from build123d import *

# Parameters (mm, degrees)
SKETCH1_W                      = 63.5
SKETCH1_H                      = 63.5
BOSS_EXTRUDE1_DEPTH            = 31.75
SKETCH2_W                      = 63.5
SKETCH2_H                      = 63.5
SKETCH2_W_2                    = 57.15
SKETCH2_H_2                    = 57.15
BOSS_EXTRUDE2_DEPTH            = 82.55
SKETCH3_W                      = 63.5
SKETCH3_H                      = 12.7
BOSS_EXTRUDE3_DEPTH            = 19.05
F_1_1_DIAMETER_HOLE2_D         = 25.4
F_1_1_DIAMETER_HOLE2_DEPTH     = 63.5
F_1_2_0_5_DIAMETER_HOLE1_D     = 12.7
F_1_2_0_5_DIAMETER_HOLE1_DEPTH = 12.7


with BuildPart() as part:
    # Sketch1 → Boss-Extrude1 (new body)
    with BuildSketch(Plane(origin=(0, 0, 0), x_dir=(1, 0, 0), z_dir=(0, 1, 0))):
        with Locations((31.75, 31.75)):
            Rectangle(SKETCH1_W, SKETCH1_H)
    extrude(amount=BOSS_EXTRUDE1_DEPTH)

    # Sketch2 → Boss-Extrude2 (add)
    with BuildSketch(Plane(origin=(0, 31.75, 0), x_dir=(1, 0, 0), z_dir=(0, 1, 0))):
        with Locations((31.75, 31.75)):
            Rectangle(SKETCH2_W, SKETCH2_H)
        with Locations((31.75, 31.75)):
            Rectangle(SKETCH2_W_2, SKETCH2_H_2, mode=Mode.SUBTRACT)
    extrude(amount=BOSS_EXTRUDE2_DEPTH)

    # Sketch3 → Boss-Extrude3 (add)
    with BuildSketch(Plane(origin=(63.5, 0, 0), x_dir=(0, 0, -1), z_dir=(1, 0, 0))):
        with Locations((31.75, 107.95)):
            Rectangle(SKETCH3_W, SKETCH3_H)
    boss_extrude3 = extrude(amount=BOSS_EXTRUDE3_DEPTH)

    # Mirror2: Boss-Extrude3 across plane
    add(boss_extrude3.mirror(Plane(origin=(31.75, 0, 0), x_dir=(0, 0, 1), z_dir=(1, 0, 0))))

    # 1 (1) Diameter Hole2
    with Locations(Plane(origin=(63.5, 0, 0), x_dir=(0, 0, -1), z_dir=(1, 0, 0))):
        with Locations((31.75, 15.875)):
            Hole(F_1_1_DIAMETER_HOLE2_D / 2, depth=F_1_1_DIAMETER_HOLE2_DEPTH)

    # 1/2 (0.5) Diameter Hole1
    with Locations(Plane(origin=(0, 114.3, 0), x_dir=(1, 0, 0), z_dir=(0, 1, 0))):
        with Locations((72.39, 31.75), (-8.89, 31.593283178)):
            Hole(F_1_2_0_5_DIAMETER_HOLE1_D / 2, depth=F_1_2_0_5_DIAMETER_HOLE1_DEPTH)


solid = part.part
Can you work these out from the model? Positions are in its coordinate system, mm. A direction names the side the tool comes from. Coordinates: 2 decimals unless noted, no trailing zeros. Write each loop counter-clockwise with the first axis right and the second up, starting at its lowest first coordinate (ties: lowest second). Pieces come first, ordered by that corner, then holes. Notation, with made-up numbers: (-27.75, 52) -> (2.25, 52) arc R34 cw to (2.25, 86) -> close; hole circle Ø8 at (69, -33). An arc over 180 degrees is marked (long way). Write item = value, one per line.
(1) For pin 1 (17 mm diameter, centred on y = 72.5, z = -42, fed in from +X); pin 2 (6 mm diameter, centred on x = 23, z = -37, fed in from -Y); pin 3 (9.5 mm diameter, centred on x = 76, z = -23, fed in from -Y); pin 4 (17 mm diameter, centred on y = 70, z = -39.5, fed in from -X), each with a flat end and sliding along its axis, tell me the tip position at first contact or that it passes through.
Verdict:
pin_1 = 63.5
pin_2 = 0
pin_3 = 101.6
pin_4 = 0
(2) If I drill on probe 1 along X at (y, z) = (47, -22) (3 decimals); probe 2 along Z at (x, y) = (72, 108); probe 3 along Z at (x, y) = (-8.89, 110.5), over which ranges is the centre line in solid material (lowest first)?
Verdict:
probe_1 = 0 to 3.175, 60.325 to 63.5
probe_2 = -63.5 to -38.09, -25.41 to 0
probe_3 = -63.5 to -37.94, -25.24 to 0
(3) Imagine slicing it at B-B (z = -49.5). Please give me the cut outline in (x, y) (3 decimals).
Verdict:
outline = (-19.05, 101.6) -> (0, 101.6) -> (0, 0) -> (63.5, 0) -> (63.5, 101.6) -> (82.55, 101.6) -> (82.55, 114.3) -> (60.325, 114.3) -> (60.325, 31.75) -> (3.175, 31.75) -> (3.175, 114.3) -> (-19.05, 114.3) -> close
(4) Imagine slicing it at A-A (x = -8.89). Please give me the cut outline in (y, z).
Verdict:
outline = (101.6, -63.5) -> (114.3, -63.5) -> (114.3, -37.94) -> (101.6, -37.94) -> close; (101.6, -25.24) -> (114.3, -25.24) -> (114.3, 0) -> (101.6, 0) -> close
(5) Thinking about a two-plate mould opening in X: for faces 1 (the face through (-7.513, 107.861, -25.394)), 2 (the face through (63.5, 50, -31)), 3 (the face through (-16, 101.6, -31)), which applies, +X half, -X half, draft (parallel to the pull), parting line (faces both ways), or undercut?
Verdict:
face_1 = undercut
face_2 = +X half
face_3 = draft
(6) On a 3-axis mill with a long thin cutter (end or side, diameter ignored), from which of +Z, -Z, +X, -X, +Y, -Y can I reach the whole of each face in a straight line? I mean faces 4 (the face through (79, 101.6, -31)), 5 (the face through (0, 50, -31)), 6 (the face through (31, 0, -32)), 7 (the face through (78.734, 107.861, -32.029)), 8 (the face through (3.175, 72, -31)). Say none if no direction works.
Verdict:
face_4 = +Z, -Z, +X, -Y
face_5 = +Z, -Z, -X, -Y
face_6 = +Z, -Z, +X, -X, -Y
face_7 = +Y, -Y
face_8 = +Y
(7) Imagine slicing it at D-D (x = 28.5). Please give me the cut outline in (y, z) (3 decimals).
Verdict:
outline = (0, -63.5) -> (114.3, -63.5) -> (114.3, -60.325) -> (31.75, -60.325) -> (31.75, -3.175) -> (114.3, -3.175) -> (114.3, 0) -> (0, 0) -> close; hole circle Ø25.4 at (15.875, -31.75)
(8) Imagine slicing it at C-C (z = -29.5). Please give me the cut outline in (x, y) (3 decimals), and give its area (3 significant figures).
Verdict:
outline = (-19.05, 101.6) -> (-14.885, 101.6) -> (-14.885, 114.3) -> (-19.05, 114.3) -> close; (-2.895, 101.6) -> (0, 101.6) -> (0, 28.374) -> (63.5, 28.374) -> (63.5, 101.6) -> (66.452, 101.6) -> (66.452, 114.3) -> (60.325, 114.3) -> (60.325, 31.75) -> (3.175, 31.75) -> (3.175, 114.3) -> (-2.895, 114.3) -> close; (0, 0) -> (63.5, 0) -> (63.5, 3.376) -> (0, 3.376) -> close; (78.328, 101.6) -> (82.55, 101.6) -> (82.55, 114.3) -> (78.328, 114.3) -> close
area = 1,130 mm^2
